Input: dimensioned drawing with shaded views. Units: mm. Origin: part minimum x, y, z. Give positions to 0.01 mm unless a question says otherwise; leave off trailing zeros. Loops run counter-clockwise (first coordinate to the right, second up) from the corner with the lowest first, then second, coordinate; pieces in that order, holes last. Notation, with made-up numbers: M 77,0 L 97,0 A20 ccw 97,25 Z; hole C 21.25,81 d10. An arc over 180 degrees is marked long. Use CSV: the item, a comma, the result in double quotes. Start each with the question number.
Q1. Material intervals for line 1 along Z through (x, y) = (85.5, 0.5) (1 decimal); line 2 along X through (y, z) = (7.25, 75); line 3 along Z through (x, y) = (70.5, 5.5), sorted ascending.
Q2. Section A-A, the plane z = 42.5. Output: boundary loops of the cut face in (x, y), plus the area to 3 significant figures.
Q3. Section B-B, the plane x = 70. Output: boundary loops of the cut face in (y, z).
Q4. Section C-C, the plane z = 10. Output: boundary loops of the cut face in (x, y), plus the area to 3 significant figures.
Q5. Section D-D, the plane y = 3.5. State how many separate pieces and enclosed holes the cut face has, plus the area to 3 significant figures.
Q6. Pin query (flat end, axial travel): pin 1 (4 mm diameter, centred on x = 55, z = 75, fed in from -Y); pin 2 (7 mm diameter, centred on x = 40, z = 10, fed in from +Y). Return the tip coordinate at first contact, or that it passes through.
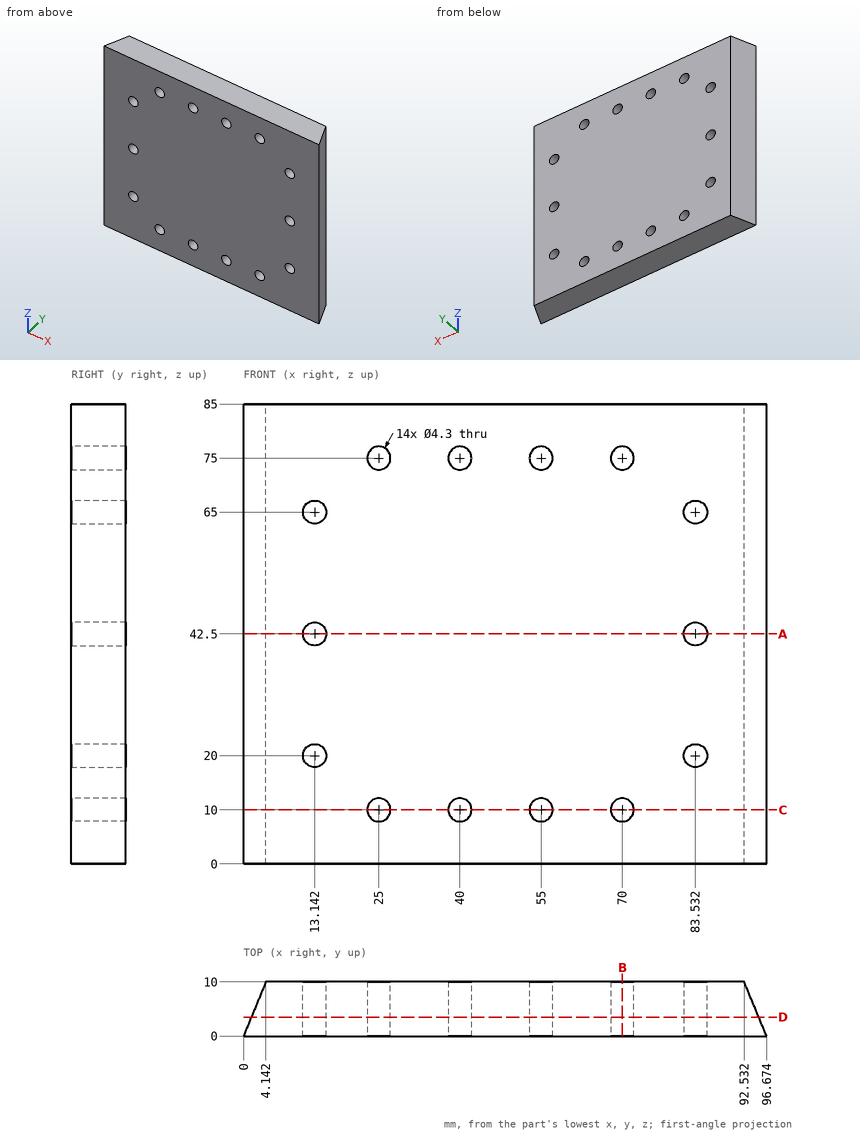
A:
1,line 1,"0 to 19.1, 20.9 to 41.6, 43.4 to 64.1, 65.9 to 85"
1,line 2,"3 to 22.85, 27.15 to 37.85, 42.15 to 52.85, 57.15 to 67.85, 72.15 to 93.67"
1,line 3,"0 to 7.91, 12.09 to 72.91, 77.09 to 85"
2,outline,"M 0,0 L 10.99,0 L 10.99,10 L 4.14,10 Z; M 15.29,0 L 81.38,0 L 81.38,10 L 15.29,10 Z; M 85.68,0 L 96.67,0 L 92.53,10 L 85.68,10 Z"
2,area,"839 mm^2"
3,outline,"M 0,0 L 10,0 L 10,7.85 L 0,7.85 Z; M 0,12.15 L 10,12.15 L 10,72.85 L 0,72.85 Z; M 0,77.15 L 10,77.15 L 10,85 L 0,85 Z"
4,outline,"M 0,0 L 22.85,0 L 22.85,10 L 4.14,10 Z; M 27.15,0 L 37.85,0 L 37.85,10 L 27.15,10 Z; M 42.15,0 L 52.85,0 L 52.85,10 L 42.15,10 Z; M 57.15,0 L 67.85,0 L 67.85,10 L 57.15,10 Z; M 72.15,0 L 96.67,0 L 92.53,10 L 72.15,10 Z"
4,area,"753 mm^2"
5,separate pieces,"1"
5,enclosed holes,"14"
5,area,"7,770 mm^2"
6,pin 1,"through"
6,pin 2,"y = 10"
